Design review of the part built by this model. Coordinates are the model's own, in mm. Coordinates: 2 decimals unless noted, no trailing zeros. Write each loop counter-clockwise with the first axis right and the second up, starting at its lowest first coordinate (ties: lowest second). Pieces come first, ordered by that corner, then holes. Notation, with made-up numbers: (81, -2.5) - (109, -2.5) arc R28 ccw to (109, 16.5) - close; hole circle Ø7 at (54.5, -26.75). An arc over 180 degrees is marked (long way). Answer as CSV lines item,"result". Start each with the question number.
Q1. We need section A-A (x = 0). Write out the cut boundary in (y, z) (3 decimals), plus the area to 3 significant figures.
Q2. Clearance check with flat-ended pins moving along their axes: pin 1 (4 mm diameter, centred on x = 0, y = -29.625, fed in from +Z); pin 2 (2.5 mm diameter, centred on x = -66.125, y = 29.625, fed in from -Z). State where each tip first meets the part, or that it passes through.
Q3. We need section D-D (z = 0.55). Write out the cut boundary in (x, y) (3 decimals).
Q4. We need section B-B (y = -4.5). Write out the cut boundary in (x, z) (3 decimals).
Q5. For line 1 along Y through (x, z) = (0, 1.05) (3 decimals); line 2 along Y through (x, z) = (47, 0.3) (3 decimals); line 3 along X through (y, z) = (20, 2.1) (3 decimals), list the stretches that pass through material, from the lowest coordinate up. Write a range as [from, to].
Q6. We need section C-C (x = -37). Write out the cut boundary in (y, z) (3 decimals), plus the area to 3 significant figures.
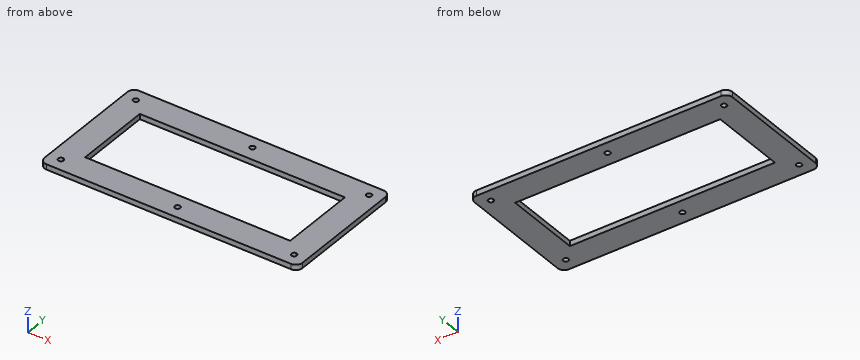
from build123d import *

# Parameters (mm, degrees)
F0_W     = 116.25
F0_H     = 43.25
F1_DEPTH = 3


with BuildPart() as f1:
    # F0 (on Top) → F1 (new body)
    with BuildSketch(Plane.XY):
        with BuildLine():
            Line((69.315, 36.625), (-69.315, 36.625))
            ThreePointArc((-69.315, 36.625), (-72.009077, 35.509077), (-73.125, 32.815))
            Line((-73.125, 32.815), (-73.125, -32.815))
            ThreePointArc((-73.125, -32.815), (-72.009077, -35.509077), (-69.315, -36.625))
            Line((-69.315, -36.625), (69.315, -36.625))
            ThreePointArc((69.315, -36.625), (72.009077, -35.509077), (73.125, -32.815))
            Line((73.125, -32.815), (73.125, 32.815))
            ThreePointArc((73.125, 32.815), (72.009077, 35.509077), (69.315, 36.625))
        make_face()
        with BuildLine():
            ThreePointArc((-66.125, 28.125), (-67.18566, 30.68566), (-64.625, 29.625))
            Line((-64.625, 29.625), (-1.5, 29.625))
            ThreePointArc((-1.5, 29.625), (0, 31.125), (1.5, 29.625))
            Line((1.5, 29.625), (64.625, 29.625))
            ThreePointArc((64.625, 29.625), (66.125, 31.125), (67.625, 29.625))
            ThreePointArc((67.625, 29.625), (67.18566, 28.56434), (66.125, 28.125))
            Line((66.125, 28.125), (66.125, -28.125))
            ThreePointArc((66.125, -28.125), (67.18566, -28.56434), (67.625, -29.625))
            ThreePointArc((67.625, -29.625), (66.125, -31.125), (64.625, -29.625))
            Line((64.625, -29.625), (1.5, -29.625))
            ThreePointArc((1.5, -29.625), (0, -31.125), (-1.5, -29.625))
            Line((-1.5, -29.625), (-64.625, -29.625))
            ThreePointArc((-64.625, -29.625), (-67.18566, -30.68566), (-66.125, -28.125))
            Line((-66.125, -28.125), (-66.125, 28.125))
        make_face(mode=Mode.SUBTRACT)
        with BuildLine():
            Line((-1.5, 29.625), (-64.625, 29.625))
            ThreePointArc((-64.625, 29.625), (-65.06434, 28.56434), (-66.125, 28.125))
            Line((-66.125, 28.125), (-66.125, -28.125))
            ThreePointArc((-66.125, -28.125), (-65.06434, -28.56434), (-64.625, -29.625))
            Line((-64.625, -29.625), (-1.5, -29.625))
            ThreePointArc((-1.5, -29.625), (0, -28.125), (1.5, -29.625))
            Line((1.5, -29.625), (64.625, -29.625))
            ThreePointArc((64.625, -29.625), (65.06434, -28.56434), (66.125, -28.125))
            Line((66.125, -28.125), (66.125, 28.125))
            ThreePointArc((66.125, 28.125), (65.06434, 28.56434), (64.625, 29.625))
            Line((64.625, 29.625), (1.5, 29.625))
            ThreePointArc((1.5, 29.625), (0, 28.125), (-1.5, 29.625))
        make_face()
        Rectangle(F0_W, F0_H, mode=Mode.SUBTRACT)
    extrude(amount=F1_DEPTH)


solid = f1.part
Results list:
1,outline,"(-36.625, 0) - (-31.125, 0) - (-31.125, 3) - (-36.625, 3) - close; (-28.125, 0) - (-21.625, 0) - (-21.625, 3) - (-28.125, 3) - close; (21.625, 0) - (28.125, 0) - (28.125, 3) - (21.625, 3) - close; (31.125, 0) - (36.625, 0) - (36.625, 3) - (31.125, 3) - close"
1,area,"72.0 mm2"
2,pin 1,"stops at z = 3"
2,pin 2,"passes through"
3,outline,"(-73.125, -32.815) arc R3.81 ccw to (-69.315, -36.625) - (69.315, -36.625) arc R3.81 ccw to (73.125, -32.815) - (73.125, 32.815) arc R3.81 ccw to (69.315, 36.625) - (-69.315, 36.625) arc R3.81 ccw to (-73.125, 32.815) - close; hole circle Ø3 at (-66.125, -29.625); hole circle Ø3 at (-66.125, 29.625); hole (-58.125, -21.625) - (58.125, -21.625) - (58.125, 21.625) - (-58.125, 21.625) - close; hole circle Ø3 at (0, -29.625); hole circle Ø3 at (0, 29.625); hole (64.625, -29.625) arc R1.5 ccw (long way) to (66.125, -28.125) arc R1.5 ccw to start; hole (66.125, 28.125) arc R1.5 ccw to (67.625, 29.625) arc R1.5 ccw (long way) to start"
4,outline,"(-73.125, 0) - (-58.125, 0) - (-58.125, 3) - (-73.125, 3) - close; (58.125, 0) - (73.125, 0) - (73.125, 3) - (58.125, 3) - close"
5,line 1,"y = [-36.625, -31.125], [-28.125, -21.625], [21.625, 28.125], [31.125, 36.625]"
5,line 2,"y = [-36.625, -21.625], [21.625, 36.625]"
5,line 3,"x = [-73.125, -58.125], [58.125, 73.125]"
6,outline,"(-36.625, 0) - (-21.625, 0) - (-21.625, 3) - (-36.625, 3) - close; (21.625, 0) - (36.625, 0) - (36.625, 3) - (21.625, 3) - close"
6,area,"90.0 mm2"
